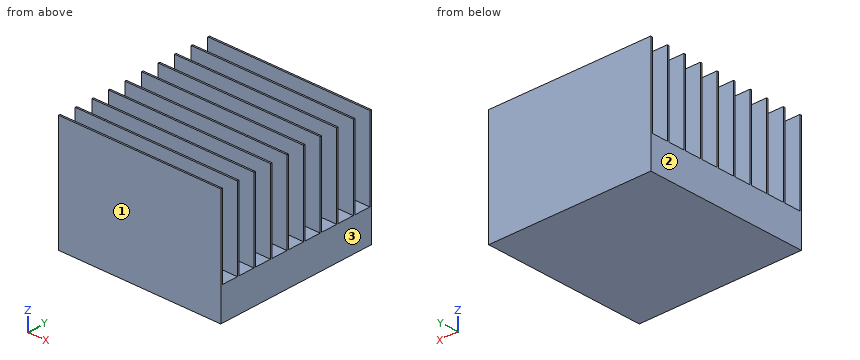
```python
from build123d import *

# Parameters (mm, degrees)
SKETCH2_W           = 25.4
SKETCH2_H           = 25.4
BOSS_EXTRUDE1_DEPTH = 5.08
SKETCH3_W           = 25.4
SKETCH3_H           = 0.254
BOSS_EXTRUDE2_DEPTH = 12.7
SKETCH6_W           = 25.4
SKETCH6_H           = 0.254
BOSS_EXTRUDE3_DEPTH = 12.5984
SKETCH5_W           = 25.4
SKETCH5_H           = 0.254
BOSS_EXTRUDE4_DEPTH = 12.7
SKETCH4_W           = 25.4
SKETCH4_H           = 0.254
BOSS_EXTRUDE5_DEPTH = 12.7


with BuildPart() as part:
    # Sketch2 → Boss-Extrude1 (new body)
    with BuildSketch(Plane.XY):
        with Locations((12.7, 12.7)):
            Rectangle(SKETCH2_W, SKETCH2_H)
    extrude(amount=BOSS_EXTRUDE1_DEPTH)

    # Sketch3 → Boss-Extrude2 (add)
    with BuildSketch(Plane.XY.offset(5.08)):
        with Locations((12.7, 25.273)):
            Rectangle(SKETCH3_W, SKETCH3_H)
    extrude(amount=BOSS_EXTRUDE2_DEPTH)

    # Sketch6 → Boss-Extrude3 (add)
    with BuildSketch(Plane.XY.offset(5.08)):
        with Locations((12.7, 11.303)):
            Rectangle(SKETCH6_W, SKETCH6_H)
        with Locations((12.7, 8.509)):
            Rectangle(SKETCH6_W, SKETCH6_H)
        with Locations((12.7, 5.715)):
            Rectangle(SKETCH6_W, SKETCH6_H)
        with Locations((12.7, 2.921)):
            Rectangle(SKETCH6_W, SKETCH6_H)
    extrude(amount=BOSS_EXTRUDE3_DEPTH)

    # Sketch5 → Boss-Extrude4 (add)
    with BuildSketch(Plane.XY.offset(5.08)):
        with Locations((12.7, 19.685)):
            Rectangle(SKETCH5_W, SKETCH5_H)
        with Locations((12.7, 16.891)):
            Rectangle(SKETCH5_W, SKETCH5_H)
        with Locations((12.7, 14.097)):
            Rectangle(SKETCH5_W, SKETCH5_H)
    extrude(amount=BOSS_EXTRUDE4_DEPTH)

    # Sketch4 → Boss-Extrude5 (add)
    with BuildSketch(Plane.XY.offset(5.08)):
        with Locations((12.7, 0.127)):
            Rectangle(SKETCH4_W, SKETCH4_H)
        with Locations((12.7, 22.479)):
            Rectangle(SKETCH4_W, SKETCH4_H)
    extrude(amount=BOSS_EXTRUDE5_DEPTH)


solid = part.part
```
Geometry: final body of the model. Coordinates: model frame, mm. Face numbers are marked on the shaded views. Round coordinates to 2 decimals unless told otherwise and drop trailing zeros. Loops run counter-clockwise (first coordinate to the right, second up) from the corner with the lowest first, then second, coordinate; pieces in that order, holes last. Notation, with made-up numbers: (-2, -27) -> (13, -27) arc R8 cw to (13, -13) -> close; hole circle Ø6 at (-28.75, -32). An arc over 180 degrees is marked (long way). Write each question's results on one line, items separated by ' | '.
Item 1: Cut plane B-B on y = 15.75. Return the cut outline in (x, z).
Answers below:
outline: (0, 0) -> (25.4, 0) -> (25.4, 5.08) -> (0, 5.08) -> close
Item 2: Cut plane A-A on z = 13. State how many separate pieces and enclosed holes the cut face has, and give its area (3 significant figures).
Answers below:
separate pieces: 10 | enclosed holes: 0 | area: 64.5 mm²
Item 3: Line query: probe 1 along Z at (x, y) = (11.5, 15.5); probe 2 along Z at (x, y) = (18.75, 8.5). Output: solid intervals per line, ascending. Write a range as [from, to].
Answers below:
probe 1: z = [0, 5.08] | probe 2: z = [0, 17.68]
Item 4: Pull-direction query (X, two-part tool) for the marked faces 1, 2 and 3; classes: pulls with the +X half, pulls with the -X half, needs draft (parallel to the pull), parting line crosses it, or undercut.
Answers below:
face 1: needs draft | face 2: pulls with the -X half | face 3: pulls with the +X half
Item 5: Pin query (flat end, axial travel): pin 1 Ø2 at (x, y) = (6.5, 10.5) entering from +Z; pin 2 Ø1.3 at (x, y) = (10.5, 18) entering from +Z. Return the tip coordinate at first contact, or that it passes through.
Answers below:
pin 1: stops at z = 17.68 | pin 2: stops at z = 5.08
